The drawing under review shows one solid part. Ordinate dimensions are in mm from its lowest x, y, z. Coordinates: 2 decimals unless noted, no trailing zeros. Write each loop counter-clockwise with the first axis right and the second up, starting at its lowest first coordinate (ties: lowest second). Pieces come first, ordered by that corner, then holes.
1) For line 1 (Y direction, x = 11, z = 5.08) (1 decimal); line 2 (X direction, y = 128, z = 5.75); line 3 (X direction, y = 47, z = 9.5), list the stretches that pass through material, from the lowest coordinate up.
2) For P1, Ø3, axis at y = 218.5, z = 3.5, coming from the -X side; P2, Ø3, axis at y = 99.5, z = 7, coming from the -X side; P3, Ø1, axis at x = 17, z = 5.5, coming from the -Y side; P4, Ø4.5, axis at y = 6.35, z = 5.08, coming from the +X side, all flat-tipped, find the tip position at first contact; note any pin that passes through.
3) Mouldability with a two-part tool opening along Y and no side actions: class the marked faces 1 and 2 as released by +Y, released by -Y, zero draft, split by the parting line, or undercut.
4) Add section A-A, the plane z = 5.08. State the section outline as (x, y) points (1 decimal).
5) Add section C-C, the plane x = 3.25. Give the number of separate pieces and of enclosed holes in the cut face, then the cut area to 3 significant figures.
6) Add section B-B, the plane y = 198.5. State the section outline as (x, z) points (1 decimal).
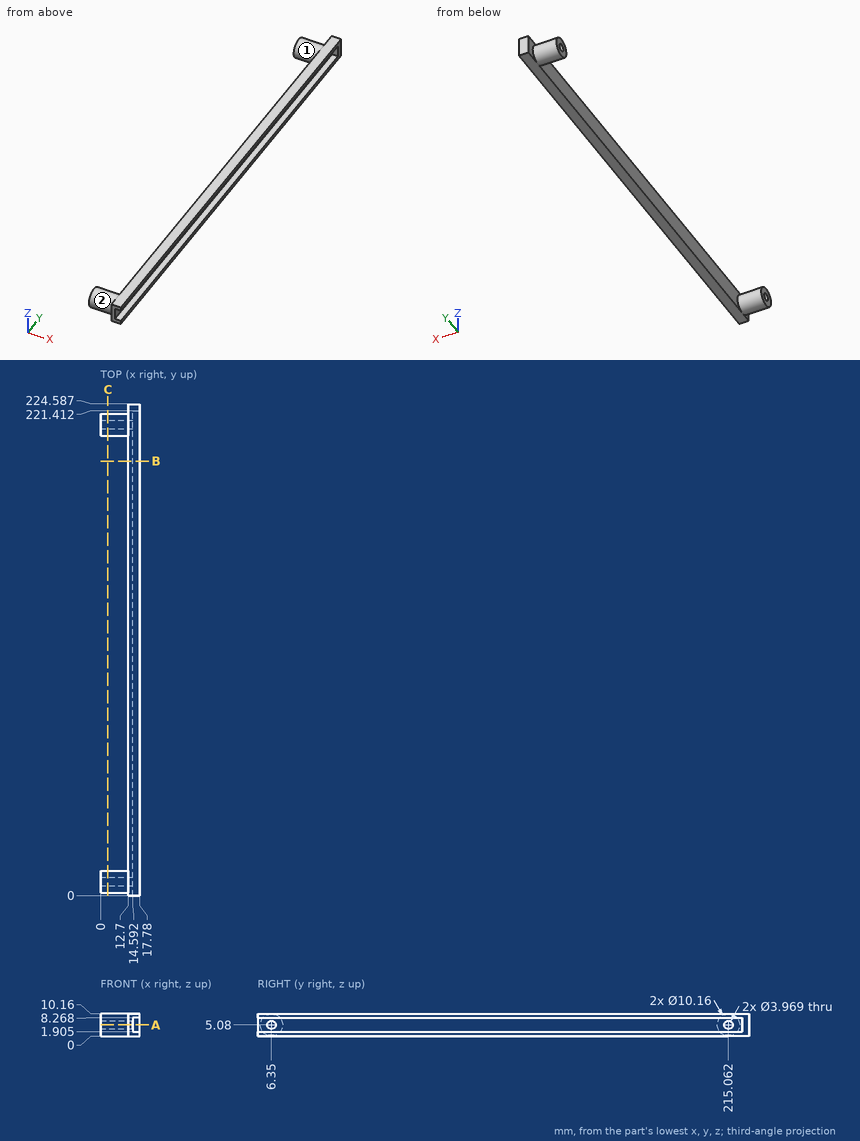
Geometry results:
1. line 1: y = 1.3 to 4.4, 8.3 to 11.4, 210 to 213.1, 217 to 220.1
1. line 2: x = 12.7 to 14.59
1. line 3: x = 12.7 to 17.78
2. P1: stops at x = 0
2. P2: stops at x = 12.7
2. P3: stops at y = 221.41
2. P4: stops at x = 14.59
3. face 1: undercut
3. face 2: undercut
4. outline: (0, 1.3) - (12.7, 1.3) - (12.7, 0) - (14.6, 0) - (14.6, 4.4) - (0, 4.4) - close; (0, 8.3) - (14.6, 8.3) - (14.6, 213.1) - (0, 213.1) - (0, 210) - (12.7, 210) - (12.7, 11.4) - (0, 11.4) - close; (0, 217) - (14.6, 217) - (14.6, 221.4) - (17.8, 221.4) - (17.8, 224.6) - (12.7, 224.6) - (12.7, 220.1) - (0, 220.1) - close
5. separate pieces: 2
5. enclosed holes: 2
5. area: 137 mm2
6. outline: (12.7, 0) - (17.8, 0) - (17.8, 1.9) - (14.6, 1.9) - (14.6, 8.3) - (17.8, 8.3) - (17.8, 10.2) - (12.7, 10.2) - close
